Input: part model. Units: mm. Frame: model coordinates. Round coordinates to 2 decimals unless told otherwise and drop trailing zeros. Loops run counter-clockwise (first coordinate to the right, second up) from the corner with the lowest first, then second, coordinate; pieces in that order, holes last. Notation, with made-up numbers: (-2.75, 28.5) -> (21.25, 28.5) arc R20 ccw to (21.25, 53.5) -> close; hole circle Ø7 at (53, -25.75). An arc over 180 degrees is marked (long way). One line per question, with ' | ' between items. Start each with the question number.
Q1. Cut plane C-C on x = 370. Return loops of the section in (y, z).
Q2. Cut plane B-B on y = 500. Return loops of the section in (x, z).
Q3. Cut plane D-D on z = -552. Return loops of the section in (x, y).
Q4. Contact query for flat-ended pins moving along their axis: P1, Ø2, axis at y = 127.5, z = -661.5, coming from the -X side; P2, Ø1, axis at x = 828.5, y = 785.5, coming from the +Z side. Output: stop coordinate, or through.
Q5. Cut plane A-A on z = -896. Return loops of the section in (x, y).
Q6. Mould query, pull axis Y, two halves, no side actions, for faces 1 (the face through (60.142, 57.032, -507)), 2 (the face through (82.085, 575.093, -738.455)), 3 (the face through (60.142, 942.968, -507)). Classes: pulls with the +Y half, pulls with the -Y half, needs draft (parallel to the pull), parting line crosses it, or undercut.
Q7. Material intervals for L1, parallel to Z at x = 42, y = 500; L2, parallel to Y at x = 405, z = -723; L3, parallel to X at y = 333, z = -817.5, sorted ascending.
from build123d import *

# Parameters (mm, degrees)
SKETCH5_W           = 1000
SKETCH5_H           = 1000
BOSS_EXTRUDE2_DEPTH = 1000
SKETCH7_R           = 250
CUT_EXTRUDE2_DEPTH  = 400
FILLET1_R           = 200


with BuildPart() as part:
    # Sketch5 → Boss-Extrude2 (new body)
    with BuildSketch(Plane(origin=(0, 0, 0), x_dir=(0, 0, -1), z_dir=(1, 0, 0))):
        with Locations((500, 500)):
            Rectangle(SKETCH5_W, SKETCH5_H)
    extrude(amount=BOSS_EXTRUDE2_DEPTH)

    # Sketch6 → Cut-Revolve5 (revolve, cut)
    with BuildSketch(Plane(origin=(500, 0, 0), x_dir=(0, 0, -1), z_dir=(1, 0, 0))):
        with BuildLine():
            Line((83.20002133, 500), (916.79997867, 500))
            ThreePointArc((916.79997867, 500), (500, 916.79997867), (83.20002133, 500))
        make_face()
    revolve(axis=Axis((500, 500, -83.20002133), (0, 0, -1)), mode=Mode.SUBTRACT)

    # Sketch7 → Cut-Extrude2 (cut)
    with BuildSketch(Plane(origin=(0, 0, 0), x_dir=(0, 0, -1), z_dir=(1, 0, 0))):
        with Locations((500, 500)):
            Circle(SKETCH7_R)
    extrude(amount=CUT_EXTRUDE2_DEPTH, mode=Mode.SUBTRACT)

    # Fillet1
    fillet1_edges = [part.edges().sort_by_distance(p)[0] for p in [
        (0, 1000, -500),
        (0, 0, -500),
    ]]
    fillet(fillet1_edges, radius=FILLET1_R)


solid = part.part
Results:
1) outline: (0, -1000) -> (1000, -1000) -> (1000, 0) -> (0, 0) -> close; hole circle Ø792.02 at (500, -500)
2) outline: (0, -1000) -> (1000, -1000) -> (1000, 0) -> (0, 0) -> (0, -250) -> (166.5, -250) arc R416.8 cw (long way) to (166.5, -750) -> (0, -750) -> close
3) outline: (0, 200) arc R200 ccw to (200, 0) -> (1000, 0) -> (1000, 1000) -> (200, 1000) arc R200 ccw to (0, 800) -> (0, 744.53) -> (166.5, 744.53) arc R413.54 cw (long way) to (166.5, 255.47) -> (0, 255.47) -> close
4) P1: x = 13.22 | P2: z = 0
5) outline: (0, 200) arc R200 ccw to (200, 0) -> (1000, 0) -> (1000, 1000) -> (200, 1000) arc R200 ccw to (0, 800) -> close; hole circle Ø260.05 at (500, 500)
6) face 1: pulls with the -Y half | face 2: undercut | face 3: pulls with the +Y half
7) L1: -1000 to -750, -250 to 0 | L2: 0 to 160.93, 839.07 to 1000 | L3: 0 to 287.8, 712.2 to 1000
